from build123d import *

# Parameters (mm, degrees)
F0_W     = 381
F0_H     = 152.4
F1_DEPTH = 12.7
F2_W     = 89.1376596271
F2_H     = 127
F3_DEPTH = 6.35
F4_R     = 5.08
F5_W     = 127
F5_H     = 101.6
F6_DEPTH = 6.35
F7_R     = 5.08
F9_D     = 5.1054


with BuildPart() as f1:
    # F0 (on Top) → F1 (new body)
    with BuildSketch(Plane.XY):
        Rectangle(F0_W, F0_H)
    extrude(amount=F1_DEPTH)

    # F2 (on face) → F3 (cut)
    with BuildSketch(Plane.XY.offset(12.7)):
        with Locations((-133.2311701864, -0.2413299241)):
            Rectangle(F2_W, F2_H)
    extrude(amount=-F3_DEPTH, mode=Mode.SUBTRACT)

    # F4
    f4_edges = [f1.edges().sort_by_distance(p)[0] for p in [
        (-177.8, 63.25867, 9.525),
        (-177.8, -63.74133, 9.525),
        (-88.66234, 63.25867, 9.525),
        (-88.66234, -63.74133, 9.525),
    ]]
    fillet(f4_edges, radius=F4_R)

    # F5 (on face) → F6 (join)
    with BuildSketch(Plane.XY.offset(12.7)):
        with Locations((76.2, 0)):
            Rectangle(F5_W, F5_H)
    extrude(amount=F6_DEPTH)

    # F7
    f7_edges = [f1.edges().sort_by_distance(p)[0] for p in [
        (12.7, -50.8, 15.875),
        (139.7, -50.8, 15.875),
        (139.7, 50.8, 15.875),
        (12.7, 50.8, 15.875),
    ]]
    fillet(f7_edges, radius=F7_R)

    # F9 (through all)
    with Locations(Plane.XY.offset(19.05)):
        with Locations((40.3518900275, 0), (96.4727550745, 0)):
            Hole(F9_D / 2)


solid = f1.part
Build history of the part. All positions in model axes, mm. A direction names the side the tool comes from. Round coordinates to 2 decimals unless told otherwise and drop trailing zeros. Write each loop counter-clockwise with the first axis right and the second up, starting at its lowest first coordinate (ties: lowest second). Pieces come first, ordered by that corner, then holes. Notation, with made-up numbers: (74.5, -34.5) -> (102.5, -34.5) arc R12 ccw to (102.5, -19.5) -> close; hole circle Ø2 at (24, 73.25). An arc over 180 degrees is marked (long way). Write item = value, one per line.
(1) Two-plate mould, pull along X, no slides. Class faces 1 (the face through (-3, 1, 0)), 2 (the face through (12.7, -1, 16)), 3 (the face through (139.7, -1, 16)), 4 (the face through (-177.8, -1, 10)): pulls with the +X half, pulls with the -X half, needs draft (parallel to the pull), parting line crosses it, or undercut.
Answer:
face_1 = needs draft
face_2 = pulls with the -X half
face_3 = pulls with the +X half
face_4 = undercut
(2) Band-saw the part on C-C (x = 24). Give the cut face in (y, z), then the cut area to 3 significant figures.
Answer:
outline = (-76.2, 0) -> (76.2, 0) -> (76.2, 12.7) -> (50.8, 12.7) -> (50.8, 19.05) -> (-50.8, 19.05) -> (-50.8, 12.7) -> (-76.2, 12.7) -> close
area = 2,580 mm2
(3) Probe L1, parallel to X at y = 21, z = 8.5; L2, parallel to Y at x = 108, z = 13.25; L3, parallel to Z at x = -6.5, y = -33.5. List the from-to ranges inside material, lowest first.
Answer:
L1 = -190.5 to -177.8, -88.66 to 190.5
L2 = -50.8 to 50.8
L3 = 0 to 12.7
(4) Band-saw the part on D-D (x = -43). Give the cut face in (y, z).
Answer:
outline = (-76.2, 0) -> (76.2, 0) -> (76.2, 12.7) -> (-76.2, 12.7) -> close
(5) Band-saw the part on A-A (x = -121). Give the cut face in (y, z), then the cut area to 3 significant figures.
Answer:
outline = (-76.2, 0) -> (76.2, 0) -> (76.2, 12.7) -> (63.26, 12.7) -> (63.26, 6.35) -> (-63.74, 6.35) -> (-63.74, 12.7) -> (-76.2, 12.7) -> close
area = 1,130 mm2
(6) Band-saw the part on B-B (y = 29). Give the cut face in (x, z).
Answer:
outline = (-190.5, 0) -> (190.5, 0) -> (190.5, 12.7) -> (139.7, 12.7) -> (139.7, 19.05) -> (12.7, 19.05) -> (12.7, 12.7) -> (-88.66, 12.7) -> (-88.66, 6.35) -> (-177.8, 6.35) -> (-177.8, 12.7) -> (-190.5, 12.7) -> close
(7) Flat gauge pins, fed straight in: pin 1 (3 mm diameter, centred on x = 40.35, y = 0, fed in from -Z); pin 2 (1.9 mm diameter, centred on y = 16.5, z = 15.5, fed in from +X); pin 3 (8 mm diameter, centred on x = -31, y = 53.5, fed in from +Z); pin 4 (8 mm diameter, centred on x = -128, y = 8, fed in from +Z). Where does each tip first touch, or does it go through?
Answer:
pin_1 = through
pin_2 = 139.7
pin_3 = 12.7
pin_4 = 6.35
(8) Tool access for faces 5 (the face through (-134, 1, 6.35)), 6 (the face through (190.5, -1, 6)), 7 (the face through (-3, -76.2, 6)), 8 (the face through (75, -50.8, 16)), 9 (the face through (75, 50.8, 16)): list every direction of +Z, -Z, +X, -X, +Y, -Y with a clear straight run to the whole face (end or side of a thin tool).
Answer:
face_5 = +Z
face_6 = +Z, -Z, +X, +Y, -Y
face_7 = +Z, -Z, +X, -X, -Y
face_8 = +Z, +X, -X, -Y
face_9 = +Z, +X, -X, +Y
